```python
from build123d import *

# Parameters (mm, degrees)
SKETCH1_W            = 30
SKETCH1_H            = 10
BOSS_EXTRUDE1_DEPTH  = 2
M3_CLEARANCE_HOLE1_D = 3.4
SKETCH5_W            = 30
SKETCH5_H            = 2
CUT_EXTRUDE1_DEPTH   = 1.6
FILLET1_R            = 2


with BuildPart() as part:
    # Sketch1 → Boss-Extrude1 (new body)
    with BuildSketch(Plane.XY):
        Rectangle(SKETCH1_W, SKETCH1_H)
    extrude(amount=BOSS_EXTRUDE1_DEPTH)

    # M3 Clearance Hole1 (through all)
    with Locations(Plane.XY.offset(2)):
        with Locations((-7, 0), (7, 0)):
            Hole(M3_CLEARANCE_HOLE1_D / 2)

    # Sketch5 → Cut-Extrude1 (cut)
    with BuildSketch(Plane(origin=(0, 5, 0), x_dir=(1, 0, 0), z_dir=(0, 1, 0))):
        with Locations((0, -1)):
            Rectangle(SKETCH5_W, SKETCH5_H)
    extrude(amount=-CUT_EXTRUDE1_DEPTH, mode=Mode.SUBTRACT)

    # Fillet1
    fillet1_edges = [part.edges().sort_by_distance(p)[0] for p in [
        (15, 3.4, 1),
        (-15, 3.4, 1),
        (15, -5, 1),
        (-15, -5, 1),
    ]]
    fillet(fillet1_edges, radius=FILLET1_R)


solid = part.part
```
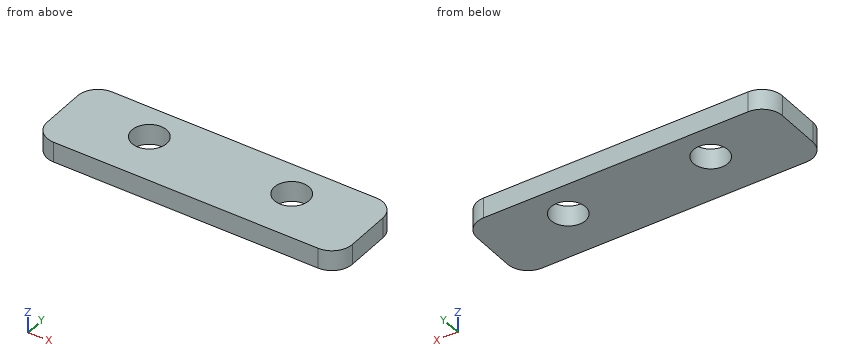
Check sheet for the modelled part. Datum: model origin and axes. Units: mm. Round coordinates to 2 decimals unless told otherwise and drop trailing zeros. Write each loop counter-clockwise with the first axis right and the second up, starting at its lowest first coordinate (ties: lowest second). Pieces come first, ordered by that corner, then holes. Notation, with made-up numbers: M 80,-12 L 136,-12 A21 cw 136,7 Z; hole C -34.75,63.25 d5. An arc over 180 degrees is marked long. Write item = value, one per line. Start each with the question number.
1. Gauge pin test, flat end, axial feed: pin 1 (1 mm diameter, centred on y = 2.5, z = 0, fed in from +X). Record the tip position at first contact, or that the pin passes through.
2. Scan lines: line 1 (X direction, y = -1.25, z = 0.6); line 2 (Y direction, x = -7, z = 0.7); line 3 (X direction, y = 0.5, z = 1.85). Record each from-to range of solid material in increasing order. Write a range as [from, to].
3. Section check A-A, the plane x = 7. Record the cut outline in (y, z).
4. Section check C-C, the plane y = 0.5. Record the cut outline in (x, z).
5. Section check B-B, the plane z = 1.3. Record the cut outline in (x, y).
Results found:
q1.pin_1 = 14.91
q2.line_1 = [-15, -8.15], [-5.85, 5.85], [8.15, 15]
q2.line_2 = [-5, -1.7], [1.7, 3.4]
q2.line_3 = [-15, -8.62], [-5.38, 5.38], [8.62, 15]
q3.outline = M -5,0 L -1.7,0 L -1.7,2 L -5,2 Z; M 1.7,0 L 3.4,0 L 3.4,2 L 1.7,2 Z
q4.outline = M -15,0 L -8.62,0 L -8.62,2 L -15,2 Z; M -5.38,0 L 5.38,0 L 5.38,2 L -5.38,2 Z; M 8.62,0 L 15,0 L 15,2 L 8.62,2 Z
q5.outline = M -15,-3 A2 ccw -13,-5 L 13,-5 A2 ccw 15,-3 L 15,1.4 A2 ccw 13,3.4 L -13,3.4 A2 ccw -15,1.4 Z; hole C -7,0 d3.4; hole C 7,0 d3.4
